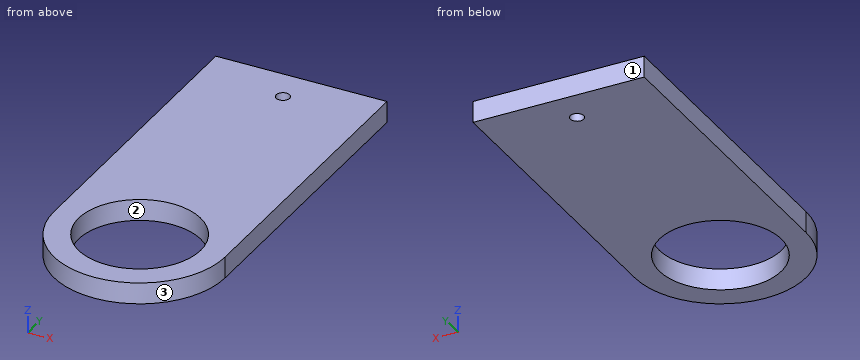
from build123d import *

# Parameters (mm, degrees)
SKETCH1_R           = 1.58
SKETCH1_R_2         = 14.26
BOSS_EXTRUDE1_DEPTH = 5


with BuildPart() as part:
    # Sketch1 → Boss-Extrude1 (new body)
    with BuildSketch(Plane.XY):
        with BuildLine():
            Line((-20, -76.707766284), (-20, -58.504148974))
            Line((-20, -58.504148974), (-20, -4.707766284))
            Line((-20, -4.707766284), (20, -4.707766284))
            Line((20, -4.707766284), (20, -76.707766284))
            ThreePointArc((20, -76.707766284), (0, -96.707766284), (-20, -76.707766284))
        make_face()
        with Locations((0, -12.911655735)):
            Circle(SKETCH1_R, mode=Mode.SUBTRACT)
        with Locations((0, -76.707766284)):
            Circle(SKETCH1_R_2, mode=Mode.SUBTRACT)
    extrude(amount=BOSS_EXTRUDE1_DEPTH)


solid = part.part
The listing builds one solid part. Answer for the finished solid, in the listing's coordinates (mm). Face numbers are marked on the shaded views. Coordinates: 2 decimals unless noted, no trailing zeros. Order: outer loops, then holes, each group sorted by start corner. A loop starts at its lowest first (then second) coordinate and runs counter-clockwise, first axis right, second up. Notation, with made-up numbers: (82, 61.25) -> (87, 61.25) arc R27 cw to (87, 82.25) -> close; hole circle Ø7 at (55.5, -17). An arc over 180 degrees is marked (long way). Answer in a Markdown table with one row per item. Add a question column.
Item 1: Find section C-C (z = 1.7). Write down the section's boundary in (x, y).
Item 2: Find the intervals of material crossed by L1, parallel to Y at x = 0, z = 2.5; L2, parallel to X at y = -79, z = 3.85; L3, parallel to Y at x = -3, z = 3.1, in increasing order. Write a range as from..to.
Item 3: Determine the mould class of the marked faces 1, 2 and 3 for opening direction Y: +Y half, -Y half, draft (parallel to the pull), parting line (faces both ways), or undercut.
Item 4: Find section A-A (x = 0). Write down the section's boundary in (y, z), then the cut area to 3 significant figures.
Item 5: Find section B-B (x = -5.5). Write down the section's boundary in (y, z).
Item 6: Find section D-D (y = -80.5). Write down the section's boundary in (x, z).
Result set:
| question | item | result |
|---|---|---|
| 1 | outline | (-20, -76.71) arc R20 ccw to (20, -76.71) -> (20, -4.71) -> (-20, -4.71) -> close; hole circle Ø28.52 at (0, -76.71); hole circle Ø3.16 at (0, -12.91) |
| 2 | L1 | y = -96.71..-90.97, -62.45..-14.49, -11.33..-4.71 |
| 2 | L2 | x = -19.87..-14.07, 14.07..19.87 |
| 2 | L3 | y = -96.48..-90.65, -62.77..-4.71 |
| 3 | face 1 | +Y half |
| 3 | face 2 | undercut |
| 3 | face 3 | -Y half |
| 4 | outline | (-96.71, 0) -> (-90.97, 0) -> (-90.97, 5) -> (-96.71, 5) -> close; (-62.45, 0) -> (-14.49, 0) -> (-14.49, 5) -> (-62.45, 5) -> close; (-11.33, 0) -> (-4.71, 0) -> (-4.71, 5) -> (-11.33, 5) -> close |
| 4 | area | 302 mm² |
| 5 | outline | (-95.94, 0) -> (-89.86, 0) -> (-89.86, 5) -> (-95.94, 5) -> close; (-63.55, 0) -> (-4.71, 0) -> (-4.71, 5) -> (-63.55, 5) -> close |
| 6 | outline | (-19.64, 0) -> (-13.75, 0) -> (-13.75, 5) -> (-19.64, 5) -> close; (13.75, 0) -> (19.64, 0) -> (19.64, 5) -> (13.75, 5) -> close |
